```python
from build123d import *

# Parameters (mm, degrees)
BOSS_EXTRUDE1_DEPTH = 12
SKETCH2_W           = 5
SKETCH2_H           = 3
CUT_EXTRUDE1_DEPTH  = 10
CUT_EXTRUDE2_REACH  = 36.801
SKETCH3_R           = 1.5


with BuildPart() as part:
    # Sketch1 → Boss-Extrude1 (new body)
    with BuildSketch(Plane.XY):
        Polygon((-9.035894855, 9.330266172), (-16.035894855, -7.469733828), (-20.035894855, -7.469733828), (-20.035894855, -11.469733828), (-18.785894855, -11.469733828), (-18.785894855, -10.469733828), (-15.785894855, -10.469733828), (-15.785894855, -16.469733828), (-12.785894855, -16.469733828), (-12.785894855, -10.469733828), (-10.785894855, -10.469733828), (-5.035894855, 3.330266172), (8.964105145, 3.330266172), (8.964105145, 9.330266172), align=None)
    boss_extrude1 = extrude(amount=BOSS_EXTRUDE1_DEPTH)

    # Sketch2 → Cut-Extrude1 (cut)
    with BuildSketch(Plane(origin=(8.964105145, 0, 0), x_dir=(0, 0, -1), z_dir=(1, 0, 0))):
        with Locations((-5.5, 4.830266172)):
            Rectangle(SKETCH2_W, SKETCH2_H)
    cut_extrude1 = extrude(amount=-CUT_EXTRUDE1_DEPTH, mode=Mode.SUBTRACT)

    # Sketch3 → Cut-Extrude2 (cut, up to next)
    with BuildSketch(Plane(origin=(0, 9.330266172, 0), x_dir=(1, 0, 0), z_dir=(0, 1, 0)), mode=Mode.PRIVATE) as cut_extrude2_sk1:
        with Locations(Location((5.964105145, -5.5, 0), (0, 0, 180))):
            Circle(SKETCH3_R)
    cut_extrude2_tool1 = extrude(cut_extrude2_sk1.sketch, amount=-CUT_EXTRUDE2_REACH, mode=Mode.PRIVATE) & part.part
    cut_extrude2 = cut_extrude2_tool1.solids().sort_by_distance((5.964105, 9.330266, 5.5))[0]
    add(cut_extrude2, mode=Mode.SUBTRACT)

    # Mirror1: Boss-Extrude1, Cut-Extrude1, Cut-Extrude2 across plane
    add(boss_extrude1.mirror(Plane(origin=(-15.785894855, -16.469733828, 12), x_dir=(0, 0, 1), z_dir=(0, 1, 0))))
    add(cut_extrude1.mirror(Plane(origin=(-15.785894855, -16.469733828, 12), x_dir=(0, 0, 1), z_dir=(0, 1, 0))), mode=Mode.SUBTRACT)
    add(cut_extrude2.mirror(Plane(origin=(-15.785894855, -16.469733828, 12), x_dir=(0, 0, 1), z_dir=(0, 1, 0))), mode=Mode.SUBTRACT)


solid = part.part
```
Read the model definition and answer for the solid it produces. Units are mm, in the model's axes. A direction names the side the tool comes from. Coordinates: 2 decimals unless noted, no trailing zeros. Loops run counter-clockwise (first coordinate to the right, second up) from the corner with the lowest first, then second, coordinate; pieces in that order, holes last.
(1) A tool of negligible diameter and unlimited length cuts with its end or side. For faces 1 (the face through (-7.951, -29.273, 5.916)), 2 (the face through (4.533, -40.791, 5.951)), 3 (the face through (-18.786, -22, 6)), 4 (the face through (-20.036, -23, 6)), 5 (the face through (4, 5, 8)), from which of +Z, -Z, +X, -X, +Y, -Y can it reach the whole face along a straight path? Write none if from no direction.
Solution:
face 1: +Z, -Z, +X
face 2: +Y, -Y
face 3: +Z, -Z
face 4: +Z, -Z, -X, +Y, -Y
face 5: +X
(2) The part is cut by section D-D (z = 1.75). Determine the outline of the cut face in (x, y).
Solution:
outline: (-20.04, -25.47) - (-16.04, -25.47) - (-9.04, -42.27) - (8.96, -42.27) - (8.96, -36.27) - (-5.04, -36.27) - (-10.79, -22.47) - (-12.79, -22.47) - (-12.79, -10.47) - (-10.79, -10.47) - (-5.04, 3.33) - (8.96, 3.33) - (8.96, 9.33) - (-9.04, 9.33) - (-16.04, -7.47) - (-20.04, -7.47) - (-20.04, -11.47) - (-18.79, -11.47) - (-18.79, -10.47) - (-15.79, -10.47) - (-15.79, -22.47) - (-18.79, -22.47) - (-18.79, -21.47) - (-20.04, -21.47) - close
(3) Consider line 1 along Y through (x, z) = (-2.75, 5.25); line 2 along Y through (x, z) = (4.25, 4.5); line 3 along X through (y, z) = (-12.5, 10.25). Determine where each line is inside the solid, lowest interval first.
Solution:
line 1: y = -42.27 to -36.27, 3.33 to 9.33
line 2: y = -42.27 to -39.27, 6.33 to 9.33
line 3: x = -15.79 to -12.79
(4) The part is cut by section C-C (z = 5.5). Count the separate pieces of the cut face and the enclosed holes in it, and give its area (3 significant figures).
Solution:
separate pieces: 3
enclosed holes: 0
area: 391 mm2
(5) The mould has two halves that part along Y. Classify faces 6 (the face through (-12.487, -33.987, 5.916)), 7 (the face through (8.964, -40, 6)), 8 (the face through (-15.786, -17, 6)), 9 (the face through (0, 9.33, 6)): released by +Y, released by -Y, zero draft, split by the parting line, or undercut.
Solution:
face 6: released by -Y
face 7: zero draft
face 8: undercut
face 9: released by +Y
(6) The part is cut by section A-A (x = 0.5). Determine the outline of the cut face in (y, z).
Solution:
outline: (-42.27, 0) - (-36.27, 0) - (-36.27, 3) - (-39.27, 3) - (-39.27, 8) - (-36.27, 8) - (-36.27, 12) - (-42.27, 12) - close; (3.33, 0) - (9.33, 0) - (9.33, 12) - (3.33, 12) - (3.33, 8) - (6.33, 8) - (6.33, 3) - (3.33, 3) - close
(7) The part is cut by section B-B (y = 4). Determine the outline of the cut face in (x, z), and give its area (3 significant figures).
Solution:
outline: (-11.26, 0) - (8.96, 0) - (8.96, 3) - (-1.04, 3) - (-1.04, 8) - (8.96, 8) - (8.96, 12) - (-11.26, 12) - close
area: 193 mm2
(8) Flat-ended cylindrical pins translate along their axes: pin 1 Ø0.9 at (x, z) = (-18, 5.5) entering from +Y; pin 2 Ø1.2 at (x, z) = (-18, 8) entering from -Y; pin 3 Ø0.9 at (y, z) = (-37, 4.5) entering from +X. Find the tip coordinate at first contact, or state that the pin passes through.
Solution:
pin 1: stops at y = -7.47
pin 2: stops at y = -25.47
pin 3: stops at x = -1.04
